```python
from build123d import *

# Parameters (mm, degrees)
SKETCH1_W           = 120
SKETCH1_H           = 12
BOSS_EXTRUDE1_DEPTH = 4
BOSS_EXTRUDE2_DEPTH = 11.2
CUT_EXTRUDE1_DEPTH  = 3


with BuildPart() as part:
    # Sketch1 → Boss-Extrude1 (new body)
    with BuildSketch(Plane.XY):
        with Locations((-3.767369491, 28.596547675)):
            Rectangle(SKETCH1_W, SKETCH1_H)
    extrude(amount=BOSS_EXTRUDE1_DEPTH)

    # Sketch2 → Boss-Extrude2 (add)
    with BuildSketch(Plane.XY.offset(4)):
        Polygon((-3.767369491, 22.596547675), (21.232630509, 22.596547675), (21.232630509, 25.596547675), (-28.767369491, 25.596547675), (-28.767369491, 22.596547675), align=None)
    extrude(amount=BOSS_EXTRUDE2_DEPTH)

    # Sketch3 → Cut-Extrude1 (cut)
    with BuildSketch(Plane(origin=(0, 25.596547675, 0), x_dir=(1, 0, 0), z_dir=(0, 1, 0))):
        with BuildLine():
            Line((7.832630509, -11.6), (7.832630509, -7.6))
            ThreePointArc((7.832630509, -7.6), (6.232630509, -6), (4.632630509, -7.6))
            Line((4.632630509, -7.6), (4.632630509, -11.6))
            ThreePointArc((4.632630509, -11.6), (6.232630509, -13.2), (7.832630509, -11.6))
        make_face()
        with BuildLine():
            Line((-15.367369491, -7.6), (-15.367369491, -11.6))
            ThreePointArc((-15.367369491, -11.6), (-13.767369491, -13.2), (-12.167369491, -11.6))
            Line((-12.167369491, -11.6), (-12.167369491, -7.6))
            ThreePointArc((-12.167369491, -7.6), (-13.767369491, -6), (-15.367369491, -7.6))
        make_face()
    extrude(amount=-CUT_EXTRUDE1_DEPTH, mode=Mode.SUBTRACT)


solid = part.part
```
Check sheet for the modelled part. Datum: model origin and axes. Units: mm. A direction names the side the tool comes from. Round coordinates to 2 decimals unless told otherwise and drop trailing zeros. Loops run counter-clockwise (first coordinate to the right, second up) from the corner with the lowest first, then second, coordinate; pieces in that order, holes last. Notation, with made-up numbers: (-11.5, 32) - (20.5, 32) arc R19 cw to (20.5, 40) - close; hole circle Ø5 at (77, -25.75). An arc over 180 degrees is marked (long way). Answer as a JSON object with one key per item and string values. Group by question number.
Q1. Set-up check for faces 5 (the face through (6.2, 24.1, 13.2)), 6 (the face through (-3, 25.597, 10)), 7 (the face through (21.233, 24, 10)): record each of +Z, -Z, +X, -X, +Y, -Y from which the full face is reachable in a straight line by a thin tool's end or side.
Q2. Gauge pin test, flat ends, axial feed: P1, Ø8, axis at x = 15.5, z = 10.5, coming from the +Y side; P2, Ø0.9, axis at y = 24.5, z = 10, coming from the +X side; P3, Ø2.5, axis at y = 24.5, z = 9.5, coming from the -X side; P4, Ø5, axis at x = -9.5, y = 25, coming from the -Z side. Record the tip position at first contact, or that the pin passes through.
Q3. Scan lines: line 1 along Z through (x, y) = (42, 32); line 2 along Y through (x, z) = (-7, 14.25). Record each from-to range of solid material in increasing order. Write a range as [from, to].
Q4. Sectioned sample at C-C, the plane x = -33. Enter the section's corners in (y, z), plus the area to 3 significant figures.
Q5. Sectioned sample at A-A, the plane z = 10.5. Enter the section's corners in (x, y), plus the area to 3 significant figures.
Q6. Sectioned sample at B-B, the plane z = 5. Enter the section's corners in (x, y).
Q7. Mould release check, pull along Z, two halves, no side actions. Record for faces 1 (the face through (-4, 24, 15.2)), 2 (the face through (-15.367, 24, 10)), 3 (the face through (-5, 22.597, 6)), 4 (the face through (-5, 29, 0)): released by +Z, released by -Z, zero draft, split by the parting line, or undercut.
Solution:
{
 "1": {"face 5": "+Y, -Y", "face 6": "+Z, +X, -X, +Y", "face 7": "+Z, +X, +Y, -Y"},
 "2": {"P1": "stops at y = 25.6", "P2": "stops at x = 21.23", "P3": "stops at x = -28.77", "P4": "stops at z = 0"},
 "3": {"line 1": "z = [0, 4]", "line 2": "y = [22.6, 25.6]"},
 "4": {"outline": "(22.6, 0) - (34.6, 0) - (34.6, 4) - (22.6, 4) - close", "area": "48.0 mm²"},
 "5": {"outline": "(-28.77, 22.6) - (-15.37, 22.6) - (-15.37, 25.6) - (-28.77, 25.6) - close; (-12.17, 22.6) - (4.63, 22.6) - (4.63, 25.6) - (-12.17, 25.6) - close; (7.83, 22.6) - (21.23, 22.6) - (21.23, 25.6) - (7.83, 25.6) - close", "area": "131 mm²"},
 "6": {"outline": "(-28.77, 22.6) - (21.23, 22.6) - (21.23, 25.6) - (-28.77, 25.6) - close"},
 "7": {"face 1": "released by +Z", "face 2": "undercut", "face 3": "zero draft", "face 4": "released by -Z"}
}
